Here's how the part is built. I have some questions about the finished solid (model axes, mm). Round coordinates to 2 decimals unless told otherwise and drop trailing zeros. One line per item, written item: value.
from build123d import *

# Parameters (mm, degrees)
GENERALSHAPE_DEPTH           = 0.8
ADDTOLERANCE_START           = -0.8
ADDTOLERANCE_DEPTH           = 1.6
BACKPLANE_DEPTH              = 71.573791169
BACKPLANE_DEPTH_BACK         = 71.573791169
RF_W                         = 3.18
RF_H                         = 4.2
CUT_EXTRUDE1_DEPTH           = 71.587392642
FILLET1_R                    = 0.5
F_0_32_0_32_DIAMETER_HOLE1_D = 0.32
FILLET2_R                    = 0.5


# Read off the part's stored shape, not the designer's step: AddTolerance
with BuildPart() as part:
    # Sketch2 → GeneralShape (new, symmetric)
    with BuildSketch(Plane(origin=(0, 0, 0), x_dir=(1, 0, 0), z_dir=(0, 1, 0))):
        Polygon((47.4, 46.4), (37, 46.4), (37, 50), (-37, 50), (-37, 46.4), (-47.4, 46.4), (-47.4, 41.5), (-50, 41.5), (-50, -38.9), (-41.5, -47.4), (41.5, -47.4), (50, -38.9), (50, 41.5), (47.4, 41.5), align=None)
    extrude(amount=GENERALSHAPE_DEPTH, both=True)

    # AddTolerance outline → AddTolerance (cut)
    with BuildSketch(Plane(origin=(0, 0, 0), x_dir=(1, 0, 0), z_dir=(0, 1, 0)).offset(ADDTOLERANCE_START)):
        Polygon((49.9, 41.4), (49.9, -39), (50, -38.9), (50, 41.5), (47.4, 41.5), (47.4, 46.4), (37, 46.4), (37, 50), (-37, 50), (-37, 46.4), (-47.4, 46.4), (-47.4, 41.5), (-50, 41.5), (-50, -38.9), (-49.9, -39), (-49.9, 41.4), (-47.3, 41.4), (-47.3, 46.3), (-36.9, 46.3), (-36.9, 49.9), (36.9, 49.9), (36.9, 46.3), (47.3, 46.3), (47.3, 41.4), align=None)
    extrude(amount=ADDTOLERANCE_DEPTH, mode=Mode.SUBTRACT)

    # Sketch4 → Backplane (cut, two sides: drawn at the far end of the back side and taken through both)
    with BuildSketch(Plane(origin=(0, 0, 0), x_dir=(1, 0, 0), z_dir=(0, 1, 0)).offset(-BACKPLANE_DEPTH_BACK)):
        with BuildLine():
            Line((41.5, -47.4), (44.1, -44.8))
            Line((44.1, -44.8), (41.232050808, -44.8))
            ThreePointArc((41.232050808, -44.8), (39.5, -43.8), (37.767949192, -44.8))
            Line((37.767949192, -44.8), (18.232050808, -44.8))
            ThreePointArc((18.232050808, -44.8), (16.5, -43.8), (14.767949192, -44.8))
            Line((14.767949192, -44.8), (-14.767949192, -44.8))
            ThreePointArc((-14.767949192, -44.8), (-16.5, -43.8), (-18.232050808, -44.8))
            Line((-18.232050808, -44.8), (-37.767949192, -44.8))
            ThreePointArc((-37.767949192, -44.8), (-39.5, -43.8), (-41.232050808, -44.8))
            Line((-41.232050808, -44.8), (-44.1, -44.8))
            Line((-44.1, -44.8), (-41.5, -47.4))
            Line((-41.5, -47.4), (41.5, -47.4))
        make_face()
    extrude(amount=BACKPLANE_DEPTH + BACKPLANE_DEPTH_BACK, mode=Mode.SUBTRACT)

    # RF → Cut-Extrude1 (cut, through all)
    with BuildSketch(Plane(origin=(0, 0.8, 0), x_dir=(1, 0, 0), z_dir=(0, 1, 0))):
        with Locations((-22, -38.7)):
            Rectangle(RF_W, RF_H)
        with Locations((-28, -38.7)):
            Rectangle(RF_W, RF_H)
        with Locations((-34, -38.7)):
            Rectangle(RF_W, RF_H)
        with BuildLine():
            Line((-18.232050808, -40.8), (-20.41, -40.8))
            Line((-20.41, -40.8), (-23.59, -40.8))
            Line((-23.59, -40.8), (-26.41, -40.8))
            Line((-26.41, -40.8), (-29.59, -40.8))
            Line((-29.59, -40.8), (-32.41, -40.8))
            Line((-32.41, -40.8), (-35.59, -40.8))
            Line((-35.59, -40.8), (-37.767949192, -40.8))
            Line((-37.767949192, -40.8), (-37.767949192, -43.8))
            Line((-37.767949192, -43.8), (-39.5, -43.8))
            ThreePointArc((-39.5, -43.8), (-38.5, -44.067949192), (-37.767949192, -44.8))
            Line((-37.767949192, -44.8), (-18.232050808, -44.8))
            ThreePointArc((-18.232050808, -44.8), (-17.5, -44.067949192), (-16.5, -43.8))
            Line((-16.5, -43.8), (-18.232050808, -43.8))
            Line((-18.232050808, -43.8), (-18.232050808, -40.8))
        make_face()
    extrude(amount=-CUT_EXTRUDE1_DEPTH, mode=Mode.SUBTRACT)

    # Fillet1
    fillet1_edges = [part.edges().sort_by_distance(p)[0] for p in [
        (-23.59, 0, 36.6),
        (-20.41, 0, 36.6),
        (-18.232050808, 0, 40.8),
        (-18.232050808, 0, 43.8),
        (-37.767949192, 0, 43.8),
        (-37.767949192, 0, 40.8),
        (-35.59, 0, 36.6),
        (-32.41, 0, 36.6),
        (-29.59, 0, 36.6),
        (-26.41, 0, 36.6),
    ]]
    fillet(fillet1_edges, radius=FILLET1_R)

    # Ø0.32 (0.32) Diameter Hole1 (through all)
    with Locations(Plane(origin=(0, 0.8, 0), x_dir=(1, 0, 0), z_dir=(0, 1, 0))):
        with Locations((-20.41, -36.6), (-23.59, -36.6), (-26.41, -36.6), (-29.59, -36.6), (-32.41, -36.6), (-35.59, -36.6)):
            Hole(F_0_32_0_32_DIAMETER_HOLE1_D / 2)

    # Fillet2
    fillet2_edges = [part.edges().sort_by_distance(p)[0] for p in [
        (47.3, 0, -41.4),
        (47.3, 0, -46.3),
        (36.9, 0, -46.3),
        (-36.9, 0, -46.3),
        (-47.3, 0, -46.3),
        (-47.3, 0, -41.4),
    ]]
    fillet(fillet2_edges, radius=FILLET2_R)


solid = part.part
Q1. If we section it at A-A, the plane y = 0.3: Give the number of separate pieces and of enclosed holes in the cut face, then the cut area to 3 significant figures.
Results list:
separate pieces: 1
enclosed holes: 6
area: 9,170 mm²
Q2. Will these pins go through, and if not, where does the flat tip stop? pin 1 (0.8 mm diameter, centred on x = 49, y = 0, fed in from -Z); pin 2 (0.8 mm diameter, centred on x = -31, y = -0.5, fed in from +Z); pin 3 (0.5 mm diameter, centred on y = 0, z = -44, fed in from -X).
Results list:
pin 1: z = -41.4
pin 2: z = 40.8
pin 3: x = -47.3
Q3. If I drill on line 1 along Z through (x, y) = (-30.5, 0.7); line 2 along Z through (x, y) = (-27, 0.15); line 3 along X through (y, z) = (0.25, -43), over which ranges is the centre line in solid material (lowest first)?
Results list:
line 1: -49.9 to 40.8
line 2: -49.9 to 36.6
line 3: -47.3 to 47.3
